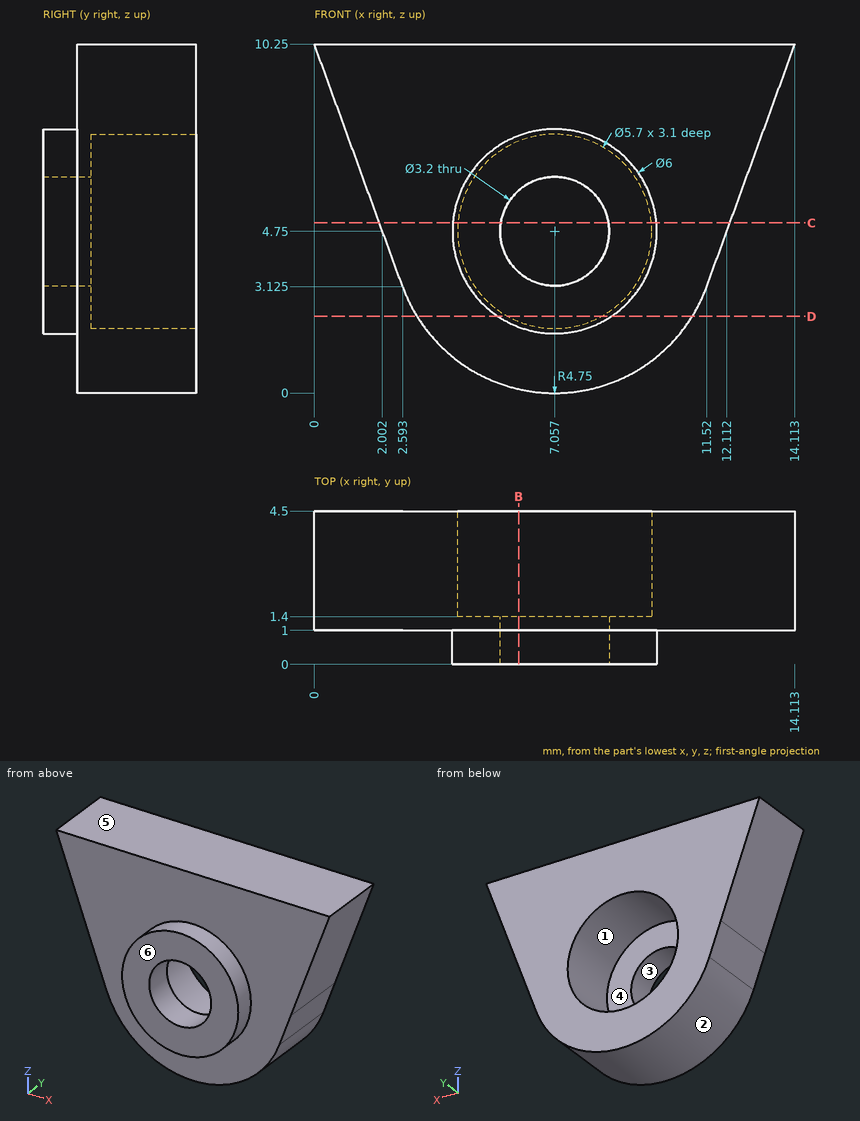
Print and shaded views of the part. All mm, measured from the part's lowest x, y and z. A direction names the side the tool comes from. Round coordinates to 2 decimals unless told otherwise and drop trailing zeros. Write each loop counter-clockwise with the first axis right and the second up, starting at its lowest first coordinate (ties: lowest second). Pieces come first, ordered by that corner, then holes.
(1) Mould opens along Z. For the marked faces 3, 4, 5 and 6 say: pulls with the +Z half, pulls with the -Z half, needs draft (parallel to the pull), parting line crosses it, or undercut.
(2) Slice it at D-D, the plane z = 2.25. Write the cut outline in (x, y) (1 decimal).
(3) Drop flat-ended pins along their axis: P1, Ø1, axis at y = 3, z = 4, coming from the -X side; P2, Ø3, axis at x = 8.5, z = 6, coming from the +Y side; P3, Ø1.9, axis at x = 7.06, z = 4.75, coming from the +Y side; P4, Ø2, axis at y = 0.5, z = 8, coming from the -X side. Give the stop position or say it passes through.
(4) Slice it at C-C, the plane z = 5. Write the cut outline in (x, y) (1 decimal).
(5) Probe line 1 along X through (y, z) = (4.15, 6.75) (1 decimal); line 2 along Y through (x, z) = (1.25, 9.5); line 3 along Z through (x, y) = (5.5, 2.5). List the from-to ranges inside material, lowest first.
(6) 3-axis set-ups, long thin cutter, end or side, ignore diameter. For the marked faces 1 and 2: which of +Z, -Z, +X, -X, +Y, -Y reach the whole face in a straight line?
(7) Slice it at B-B, the plane x = 6. Write the cut outline in (y, z).
From the geometry:
1. face 3: undercut
1. face 4: undercut
1. face 5: pulls with the +Z half
1. face 6: needs draft
2. outline: (3, 1) - (5.4, 1) - (5.4, 0) - (8.7, 0) - (8.7, 1) - (11.1, 1) - (11.1, 4.5) - (8.4, 4.5) - (8.4, 1.4) - (5.7, 1.4) - (5.7, 4.5) - (3, 4.5) - close
3. P1: stops at x = 2.09
3. P2: stops at y = 4.5
3. P3: passes through
3. P4: stops at x = 0.5
4. outline: (1.9, 1) - (4.1, 1) - (4.1, 0) - (5.5, 0) - (5.5, 1.4) - (4.2, 1.4) - (4.2, 4.5) - (1.9, 4.5) - close; (8.6, 0) - (10, 0) - (10, 1) - (12.2, 1) - (12.2, 4.5) - (9.9, 4.5) - (9.9, 1.4) - (8.6, 1.4) - close
5. line 1: x = 1.3 to 5, 9.1 to 12.8
5. line 2: y = 1 to 4.5
5. line 3: z = 0.26 to 2.36, 7.14 to 10.25
6. face 1: +Y
6. face 2: -Z, +Y, -Y
7. outline: (0, 1.94) - (1, 1.94) - (1, 0.12) - (4.5, 0.12) - (4.5, 2.1) - (1.4, 2.1) - (1.4, 3.55) - (0, 3.55) - close; (0, 5.95) - (1.4, 5.95) - (1.4, 7.4) - (4.5, 7.4) - (4.5, 10.25) - (1, 10.25) - (1, 7.56) - (0, 7.56) - close
